from build123d import *

# Parameters (mm, degrees)
SKETCH_1_R          = 2.1
SKETCH_1_R_2        = 1.6
EXTRUDE_2_DEPTH     = 8
SKETCH_3_R          = 3
SKETCH_3_R_2        = 3.5
CUT_EXTRUDE_2_DEPTH = 4
CUT_EXTRUDE_3_DEPTH = 14


with BuildPart() as part:
    # 草图1 → 凸台-拉伸2 (new body)
    with BuildSketch(Plane(origin=(0, 0, 0), x_dir=(1, 0, 0), z_dir=(0, 1, 0))):
        with BuildLine():
            Line((0, -15), (150, -15))
            ThreePointArc((150, -15), (165, 0), (150, 15))
            Line((150, 15), (0, 15))
            ThreePointArc((0, 15), (-15, 0), (0, -15))
        make_face()
        with Locations(Location((150, -9.75, 0), (0, 0, 270))):
            Circle(SKETCH_1_R, mode=Mode.SUBTRACT)
        with Locations(Location((150, 9.75, 0), (0, 0, 270))):
            Circle(SKETCH_1_R, mode=Mode.SUBTRACT)
        with Locations(Location((0, 9.75, 0), (0, 0, 270))):
            Circle(SKETCH_1_R, mode=Mode.SUBTRACT)
        with Locations(Location((0, -9.75, 0), (0, 0, 270))):
            Circle(SKETCH_1_R, mode=Mode.SUBTRACT)
        with Locations(Location((-9.75, 0, 0), (0, 0, 270))):
            Circle(SKETCH_1_R_2, mode=Mode.SUBTRACT)
        with Locations(Location((9.710485561, 0, 0), (0, 0, 270))):
            Circle(SKETCH_1_R_2, mode=Mode.SUBTRACT)
        with Locations(Location((150, 0, 0), (0, 0, 270))):
            Circle(SKETCH_1_R_2, mode=Mode.SUBTRACT)
        with Locations(Location((0, 0, 0), (0, 0, 270))):
            Circle(SKETCH_1_R_2, mode=Mode.SUBTRACT)
        with Locations(Location((159.75, 0, 0), (0, 0, 270))):
            Circle(SKETCH_1_R_2, mode=Mode.SUBTRACT)
        with Locations(Location((140.289514439, 0, 0), (0, 0, 270))):
            Circle(SKETCH_1_R_2, mode=Mode.SUBTRACT)
    extrude(amount=EXTRUDE_2_DEPTH)

    # 草图3 → 切除-拉伸2 (cut)
    with BuildSketch(Plane(origin=(0, 8, 0), x_dir=(1, 0, 0), z_dir=(0, 1, 0))):
        with Locations(Location((0, 0, 0), (0, 0, 270))):
            Circle(SKETCH_3_R)
        with Locations(Location((0, 9.75, 0), (0, 0, 270))):
            Circle(SKETCH_3_R_2)
        with Locations(Location((9.75, 0, 0), (0, 0, 270))):
            Circle(SKETCH_3_R_2)
        with Locations(Location((0, -9.75, 0), (0, 0, 270))):
            Circle(SKETCH_3_R_2)
        with Locations(Location((-9.75, 0, 0), (0, 0, 270))):
            Circle(SKETCH_3_R_2)
        with Locations(Location((159.75, 0, 0), (0, 0, 90))):
            Circle(SKETCH_3_R_2)
        with Locations(Location((150, -9.75, 0), (0, 0, 90))):
            Circle(SKETCH_3_R_2)
        with Locations(Location((140.25, 0, 0), (0, 0, 90))):
            Circle(SKETCH_3_R_2)
        with Locations(Location((150, 9.75, 0), (0, 0, 90))):
            Circle(SKETCH_3_R_2)
        with Locations(Location((150, 0, 0), (0, 0, 90))):
            Circle(SKETCH_3_R)
    extrude(amount=-CUT_EXTRUDE_2_DEPTH, mode=Mode.SUBTRACT)

    # 草图4 → 切除-拉伸3 (cut)
    with BuildSketch(Plane(origin=(0, 8, 0), x_dir=(1, 0, 0), z_dir=(0, 1, 0))):
        with BuildLine():
            Line((25, 4), (125, 4))
            ThreePointArc((125, 4), (129, 0), (125, -4))
            Line((125, -4), (25, -4))
            ThreePointArc((25, -4), (21, 0), (25, 4))
        make_face()
    extrude(amount=-CUT_EXTRUDE_3_DEPTH, mode=Mode.SUBTRACT)


solid = part.part
Geometry: final body of the model. Coordinates: model frame, mm. A direction names the side the tool comes from. Coordinates: 2 decimals unless noted, no trailing zeros. Order: outer loops, then holes, each group sorted by start corner. A loop starts at its lowest first (then second) coordinate and runs counter-clockwise, first axis right, second up. Notation, with made-up numbers: (-26, -25.5) - (-6, -25.5) arc R33 cw to (-6, 6.5) - close; hole circle Ø2 at (7.25, 45). An arc over 180 degrees is marked (long way). Use one line per item in the form item = value.
1) Ray query, L1, parallel to Z at x = 0, y = 2.55; L2, parallel to Z at x = 38.5, y = 2.5; L3, parallel to X at y = 5, z = 9. Return the intervals inside material, ascending.
Solutions:
L1 = -15 to -11.85, -7.65 to -1.6, 1.6 to 7.65, 11.85 to 15
L2 = -15 to -4, 4 to 15
L3 = -12 to -3.42, 3.42 to 146.58, 153.42 to 162
2) Section D-D (x = -9.75). Return loops of the section in (y, z).
Solutions:
outline = (0, -11.4) - (8, -11.4) - (8, -3.5) - (4, -3.5) - (4, -1.6) - (0, -1.6) - close; (0, 1.6) - (4, 1.6) - (4, 3.5) - (8, 3.5) - (8, 11.4) - (0, 11.4) - close
3) Mould query, pull axis X, two halves, no side actions, for faces 4 (the face through (165, 4, 0)), 5 (the face through (8, 4, 1)), 6 (the face through (148.44, 1.97, -0.35)), 7 (the face through (-15, 4, 0)). Classes: +X half, -X half, draft (parallel to the pull), parting line (faces both ways), or undercut.
Solutions:
face_4 = +X half
face_5 = undercut
face_6 = undercut
face_7 = -X half
4) Section C-C (y = 1.5). State how many separate pieces and enclosed holes the cut face has, then the cut area to 3 significant figures.
Solutions:
separate_pieces = 1
enclosed_holes = 11
area = 4,250 mm^2
5) Pin query (flat end, axial travel): pin 1 (5 mm diameter, centred on x = 0, z = 0, fed in from +Y); pin 2 (2 mm diameter, centred on y = 2, z = 7, fed in from +X); pin 3 (1.9 mm diameter, centred on x = 150, z = 0, fed in from -Y). Return the tip coordinate at first contact, or that it passes through.
Solutions:
pin_1 = 4
pin_2 = 163.75
pin_3 = through
6) Set-up query: faces 1 (the face through (76, 4, -15)), 2 (the face through (21, 4, 0)), 3 (the face through (-2, 4, -8)). Return all of +Z, -Z, +X, -X, +Y, -Y with unobstructed straight access to the full face (end or side cutting, diameter ignored); none if empty.
Solutions:
face_1 = -Z, +X, -X, +Y, -Y
face_2 = +Y, -Y
face_3 = +Y
7) Section A-A (x = 106.5). Return loops of the section in (y, z), then the cut area to 3 significant figures.
Solutions:
outline = (0, -15) - (8, -15) - (8, -4) - (0, -4) - close; (0, 4) - (8, 4) - (8, 15) - (0, 15) - close
area = 176 mm^2
8) Section B-B (z = 9.75). Return loops of the section in (x, y).
Solutions:
outline = (-11.4, 0) - (-2.1, 0) - (-2.1, 4) - (-3.5, 4) - (-3.5, 8) - (-11.4, 8) - close; (2.1, 0) - (147.9, 0) - (147.9, 4) - (146.5, 4) - (146.5, 8) - (3.5, 8) - (3.5, 4) - (2.1, 4) - close; (152.1, 0) - (161.4, 0) - (161.4, 8) - (153.5, 8) - (153.5, 4) - (152.1, 4) - close
